CAD build for the part. Positions are in the model's coordinates, mm. A direction names the side the tool comes from. Coordinates: 2 decimals unless noted, no trailing zeros. Order: outer loops, then holes, each group sorted by start corner. A loop starts at its lowest first (then second) coordinate and runs counter-clockwise, first axis right, second up. Notation, with made-up numbers: (2.5, -36.75) - (30.5, -36.75) arc R7 ccw to (30.5, -25.75) - close; hole circle Ø6 at (-25.75, 28.5). An arc over 180 degrees is marked (long way). Use one line per item in the form item = value.
```python
from build123d import *

# Parameters (mm, degrees)
F1_DEPTH = 6.35
F2_R     = 3.175
F3_DEPTH = 1.5885
F4_R     = 3.175
F5_DEPTH = 1.5885


with BuildPart() as f1:
    # F0 (on Front) → F1 (new body, symmetric)
    with BuildSketch(Plane.XZ):
        with BuildLine():
            Line((1.5875, 25.4), (0, 25.4))
            Line((0, 25.4), (0, 3.175))
            ThreePointArc((0, 3.175), (0.929936, 0.929936), (3.175, 0))
            Line((3.175, 0), (25.4, 0))
            Line((25.4, 0), (25.4, 1.5875))
            Line((25.4, 1.5875), (4.7625, 1.5875))
            ThreePointArc((4.7625, 1.5875), (2.517436, 2.517436), (1.5875, 4.7625))
            Line((1.5875, 4.7625), (1.5875, 25.4))
        make_face()
    extrude(amount=F1_DEPTH, both=True)

    # F2 (on face) → F3 (cut, through all)
    with BuildSketch(Plane.YZ.offset(1.5875)):
        with Locations((0, 16.523208)):
            Circle(F2_R)
    extrude(amount=-F3_DEPTH, mode=Mode.SUBTRACT)

    # F4 (on face) → F5 (cut, through all)
    with BuildSketch(Plane.XY.offset(1.5875)):
        with Locations((16.5354, 0)):
            Circle(F4_R)
    extrude(amount=-F5_DEPTH, mode=Mode.SUBTRACT)


solid = f1.part
```
Item 1: Cut at C-C, the plane z = 14.25. Write the cut outline in (x, y), plus the area to 3 significant figures.
Derived:
outline = (0, -6.35) - (1.59, -6.35) - (1.59, -2.22) - (0, -2.22) - close; (0, 2.22) - (1.59, 2.22) - (1.59, 6.35) - (0, 6.35) - close
area = 13.1 mm²
Item 2: 3-axis set-ups, long thin cutter, end or side, ignore diameter. For faces 1 (the face through (13, 0, 1.588)), 2 (the face through (13.363, 0.14, 0.805)): which of +Z, -Z, +X, -X, +Y, -Y reach the whole face in a straight line?
Derived:
face_1 = +Z, +X, +Y, -Y
face_2 = +Z, -Z
Item 3: Drop a flat-ended pin along its axis: pin 1 (3 mm diameter, centred on x = 17.5, y = 1.5, fed in from +Z). Give the stop position or say it passes through.
Derived:
pin_1 = 1.59
Item 4: Drill centre lines: line 1 (X direction, y = -1, z = 10); line 2 (Z direction, x = 1, y = 0). Where is each one in solid material? Low to high. Write a range as [from, to].
Derived:
line_1 = [0, 1.59]
line_2 = [0.86, 13.35], [19.7, 25.4]
Item 5: Two-plate mould, pull along Z, no slides. Class faces 3 (the face through (0.91, -0.09, 0.95)), 4 (the face through (1, 6.35, 7)), 5 (the face through (0.8, -0.41, 19.67)): +Z half, -Z half, draft (parallel to the pull), parting line (faces both ways), or undercut.
Derived:
face_3 = -Z half
face_4 = draft
face_5 = undercut
Item 6: Cut at B-B, the plane x = 13.75. Write the cut outline in (y, z).
Derived:
outline = (-6.35, 0) - (-1.52, 0) - (-1.52, 1.59) - (-6.35, 1.59) - close; (1.52, 0) - (6.35, 0) - (6.35, 1.59) - (1.52, 1.59) - close
Item 7: Cut at A-A, the plane y = 0. State how many separate pieces and enclosed holes the cut face has, plus the area to 3 significant figures.
Derived:
separate_pieces = 3
enclosed_holes = 0
area = 58.0 mm²
